from build123d import *

# Parameters (mm, degrees)
SKETCH1_W           = 60
SKETCH1_H           = 60
BOSS_EXTRUDE1_DEPTH = 10
SKETCH2_R           = 18.034
CUT_EXTRUDE1_DEPTH  = 86.440037453
SKETCH4_W           = 5
SKETCH4_H           = 60
BOSS_EXTRUDE2_DEPTH = 10
SKETCH5_R           = 2
CUT_EXTRUDE3_DEPTH  = 86.440037453
CAVITY3_OUTLINE_R   = 2.5
CAVITY3_DEPTH       = 5
SKETCH7_R           = 2
CUT_EXTRUDE4_DEPTH  = 88.177978871


# Read off the part's stored shape, not the designer's step: Cavity3
with BuildPart() as part:
    # Sketch1 → Boss-Extrude1 (new body)
    with BuildSketch(Plane.XY):
        with Locations((30, 30)):
            Rectangle(SKETCH1_W, SKETCH1_H)
    extrude(amount=BOSS_EXTRUDE1_DEPTH)

    # Sketch2 → Cut-Extrude1 (cut, through all)
    with BuildSketch(Plane(origin=(0, 0, 0), x_dir=(-1, 0, 0), z_dir=(0, 0, -1))):
        with Locations((-30, 30)):
            Circle(SKETCH2_R)
    extrude(amount=-CUT_EXTRUDE1_DEPTH, mode=Mode.SUBTRACT)

    # Sketch4 → Boss-Extrude2 (add)
    with BuildSketch(Plane(origin=(0, 0, 0), x_dir=(-1, 0, 0), z_dir=(0, 0, -1))):
        with Locations((-2.5, 30)):
            Rectangle(SKETCH4_W, SKETCH4_H)
    extrude(amount=BOSS_EXTRUDE2_DEPTH)

    # Sketch5 → Cut-Extrude3 (cut, through all)
    with BuildSketch(Plane.ZY):
        with Locations((-6, 50)):
            Circle(SKETCH5_R)
        with Locations((-6, 10)):
            Circle(SKETCH5_R)
    extrude(amount=-CUT_EXTRUDE3_DEPTH, mode=Mode.SUBTRACT)

    # Cavity3 outline → Cavity3 (cut)
    with BuildSketch(Plane.XY):
        with Locations((10, 10)):
            Circle(CAVITY3_OUTLINE_R)
        with Locations((50, 50)):
            Circle(CAVITY3_OUTLINE_R)
    extrude(amount=CAVITY3_DEPTH, mode=Mode.SUBTRACT)

    # Sketch7 → Cut-Extrude4 (cut, through all)
    with BuildSketch(Plane.XY.offset(10)):
        with Locations((10, 50)):
            Circle(SKETCH7_R)
        with Locations((50, 10)):
            Circle(SKETCH7_R)
    extrude(amount=-CUT_EXTRUDE4_DEPTH, mode=Mode.SUBTRACT)


solid = part.part
For this review, take the finished solid that the model builds, in its own axes (mm). A direction names the side the tool comes from. Give positions to 0.01 mm unless a question says otherwise; leave off trailing zeros. Order: outer loops, then holes, each group sorted by start corner. A loop starts at its lowest first (then second) coordinate and runs counter-clockwise, first axis right, second up. Notation, with made-up numbers: (76, 41) - (134, 41) arc R7 ccw to (134, 48) - close; hole circle Ø4 at (-21.75, 55.25). An arc over 180 degrees is marked (long way). Answer as a JSON object with one key per item and string values. Group by question number.
Item 1: Clearance check with flat-ended pins moving along their axes: pin 1 Ø5 at (y, z) = (10, -6) entering from +X; pin 2 Ø8 at (y, z) = (40.5, -3.5) entering from +X; pin 3 Ø4.5 at (x, y) = (50, 10) entering from -Z; pin 4 Ø3 at (x, y) = (50, 50) entering from -Z. State where each tip first meets the part, or that it passes through.
Item 2: Wall thickness on line 1 along Y through (x, z) = (10, 3.25); line 2 along Y through (x, z) = (49, 0.5); line 3 along Y through (x, z) = (10, 7.75): over which ranges is each line inside the solid? List them lowest first.
Item 3: Take a section at C-C on z = 7. Give the boundary of the cut face in (x, y), and give its area (3 significant figures).
Item 4: Take a section at A-A on x = 50. Give the boundary of the cut face in (y, z).
Item 5: Take a section at B-B on y = 30. Give the boundary of the cut face in (x, z).
Item 6: Take a section at D-D on z = -6. Give the boundary of the cut face in (x, y), and give its area (3 significant figures).
Item 7: Draft analysis for pull direction Y (two halves, no side actions). For faces 1 (the cylindrical face through (2.465, 48.226, -5.077)), 2 (the flat face through (50, 50, 5)), 3 (the flat face through (60, 30, 5)), 4 (the flat face through (30, 60, 5)), state which applies: pulls with the +Y half, pulls with the -Y half, needs draft (parallel to the pull), parting line crosses it, or undercut.
Item 8: Machinability: for faces 5 (the cylindrical face through (10.923, 48.226, 5.07)), 6 (the flat face through (5, 30, -5)), 7 (the cylindrical face through (52.31, 49.04, 2.46)), which of the approach directions +Z, -Z, +X, -X, +Y, -Y give a long, thin tool a straight path to every point of the face, cutting with its end or side? Answer none if there is none.
Reported:
{
 "1": {"pin 1": "x = 5", "pin 2": "x = 60", "pin 3": "z = 0", "pin 4": "z = 5"},
 "2": {"line 1": "0 to 7.5, 12.5 to 48, 52 to 60", "line 2": "0 to 8.27, 11.73 to 47.71, 52.29 to 60", "line 3": "0 to 48, 52 to 60"},
 "3": {"outline": "(0, 0) - (60, 0) - (60, 60) - (0, 60) - close; hole circle Ø4 at (10, 50); hole circle Ø36.07 at (30, 30); hole circle Ø4 at (50, 10)", "area": "2,550 mm^2"},
 "4": {"outline": "(0, 0) - (8, 0) - (8, 10) - (0, 10) - close; (12, 0) - (47.5, 0) - (47.5, 5) - (52.5, 5) - (52.5, 0) - (60, 0) - (60, 10) - (12, 10) - close"},
 "5": {"outline": "(0, -10) - (5, -10) - (5, 0) - (11.97, 0) - (11.97, 10) - (0, 10) - close; (48.03, 0) - (60, 0) - (60, 10) - (48.03, 10) - close"},
 "6": {"outline": "(0, 0) - (5, 0) - (5, 8) - (0, 8) - close; (0, 12) - (5, 12) - (5, 48) - (0, 48) - close; (0, 52) - (5, 52) - (5, 60) - (0, 60) - close", "area": "260 mm^2"},
 "7": {"face 1": "undercut", "face 2": "undercut", "face 3": "needs draft", "face 4": "pulls with the +Y half"},
 "8": {"face 5": "+Z, -Z", "face 6": "-Z, +X, +Y, -Y", "face 7": "-Z"}
}
